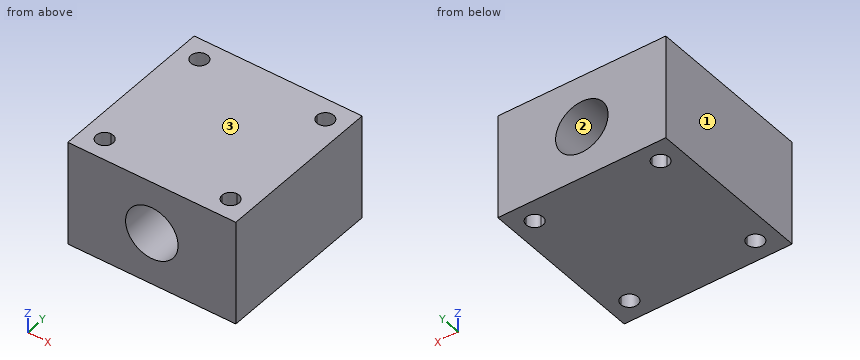
```python
from build123d import *

# Parameters (mm, degrees)
SKETCH1_W           = 80
SKETCH1_H           = 50
BOSS_EXTRUDE1_DEPTH = 80
SKETCH2_R           = 12.5
CUT_EXTRUDE1_DEPTH  = 93.870878105
CUT_EXTRUDE2_DEPTH  = 103.46950766


with BuildPart() as part:
    # Sketch1 → Boss-Extrude1 (new body)
    with BuildSketch(Plane(origin=(0, 0, 0), x_dir=(1, 0, 0), z_dir=(0, 1, 0))):
        Rectangle(SKETCH1_W, SKETCH1_H)
    extrude(amount=BOSS_EXTRUDE1_DEPTH)

    # Sketch2 → Cut-Extrude1 (cut, through all)
    with BuildSketch(Plane(origin=(0, 80, 0), x_dir=(1, 0, 0), z_dir=(0, 1, 0))):
        with Locations(Location((0, 0, 0), (0, 0, 270))):
            Circle(SKETCH2_R)
    extrude(amount=-CUT_EXTRUDE1_DEPTH, mode=Mode.SUBTRACT)

    # Sketch3 → Cut-Extrude2 (cut, through all)
    with BuildSketch(Plane.XY.offset(25)):
        with BuildLine():
            ThreePointArc((-26, 70), (-32.828427125, 72.828427125), (-30, 66))
            Line((-30, 66), (-30, 70))
            Line((-30, 70), (-26, 70))
        make_face()
        with BuildLine():
            Line((-30, 70), (-30, 66))
            ThreePointArc((-30, 66), (-27.171572875, 67.171572875), (-26, 70))
            Line((-26, 70), (-30, 70))
        make_face()
        with BuildLine():
            ThreePointArc((-30, 14), (-32.828427125, 7.171572875), (-26, 10))
            Line((-26, 10), (-30, 10))
            Line((-30, 10), (-30, 14))
        make_face()
        with BuildLine():
            Line((-30, 10), (-26, 10))
            ThreePointArc((-26, 10), (-27.171572875, 12.828427125), (-30, 14))
            Line((-30, 14), (-30, 10))
        make_face()
        with BuildLine():
            ThreePointArc((30, 14), (27.171572875, 12.828427125), (26, 10))
            Line((26, 10), (30, 10))
            Line((30, 10), (30, 14))
        make_face()
        with BuildLine():
            Line((30, 10), (26, 10))
            ThreePointArc((26, 10), (30, 6), (34, 10))
            ThreePointArc((34, 10), (32.828427125, 12.828427125), (30, 14))
            Line((30, 14), (30, 10))
        make_face()
        with BuildLine():
            ThreePointArc((26, 70), (27.171572875, 67.171572875), (30, 66))
            Line((30, 66), (30, 70))
            Line((30, 70), (26, 70))
        make_face()
        with BuildLine():
            Line((30, 70), (30, 66))
            ThreePointArc((30, 66), (32.828427125, 67.171572875), (34, 70))
            ThreePointArc((34, 70), (30, 74), (26, 70))
            Line((26, 70), (30, 70))
        make_face()
    extrude(amount=-CUT_EXTRUDE2_DEPTH, mode=Mode.SUBTRACT)


solid = part.part
```
Source: CAD feature listing. Evaluate the final solid. Frame: model axes, mm. Face numbers are marked on the shaded views. Give positions to 0.01 mm unless a question says otherwise; leave off trailing zeros. Write each loop counter-clockwise with the first axis right and the second up, starting at its lowest first coordinate (ties: lowest second). Pieces come first, ordered by that corner, then holes.
1. Section query B-B (x = 0). Return the cut outline in (y, z).
2. First-contact query: pin 1 (5 mm diameter, centred on x = -30, y = 70, fed in from -Z). Flat tip, straight axial feed; report the tip coordinate or a pass-through.
3. Section query C-C (z = 20.5). Return the cut outline in (x, y), then the cut area to 3 significant figures.
4. Pull-direction query (X, two-part tool) for the marked faces 1, 2 and 3; classes: +X half, -X half, draft (parallel to the pull), parting line (faces both ways), or undercut.
5. Section query D-D (x = 28.5). Return the cut outline in (y, z).
6. Material intervals for line 1 along Y through (x, z) = (-30, -9); line 2 along X through (y, z) = (70, -0.5); line 3 along X through (y, z) = (23, 0), sorted ascending.
7. Section query A-A (z = -0.5). Return the cut outline in (x, y), then the cut area to 3 significant figures.
Output values:
1. outline: (0, -25) - (80, -25) - (80, -12.5) - (0, -12.5) - close; (0, 12.5) - (80, 12.5) - (80, 25) - (0, 25) - close
2. pin 1: passes through
3. outline: (-40, 0) - (40, 0) - (40, 80) - (-40, 80) - close; hole circle Ø8 at (-30, 10); hole circle Ø8 at (-30, 70); hole circle Ø8 at (30, 10); hole circle Ø8 at (30, 70)
3. area: 6,200 mm2
4. face 1: -X half
4. face 2: undercut
4. face 3: draft
5. outline: (0, -25) - (6.29, -25) - (6.29, 25) - (0, 25) - close; (13.71, -25) - (66.29, -25) - (66.29, 25) - (13.71, 25) - close; (73.71, -25) - (80, -25) - (80, 25) - (73.71, 25) - close
6. line 1: y = 0 to 6, 14 to 66, 74 to 80
6. line 2: x = -40 to -34, -26 to -12.49, 12.49 to 26, 34 to 40
6. line 3: x = -40 to -12.5, 12.5 to 40
7. outline: (-40, 0) - (-12.49, 0) - (-12.49, 80) - (-40, 80) - close; (12.49, 0) - (40, 0) - (40, 80) - (12.49, 80) - close; hole circle Ø8 at (-30, 10); hole circle Ø8 at (-30, 70); hole circle Ø8 at (30, 10); hole circle Ø8 at (30, 70)
7. area: 4,200 mm2
